from build123d import *

# Parameters (mm, degrees)
F0_W           = 177.8
F0_H           = 228.6
F1_DEPTH       = 12.7
F2_R           = 38.1
F3_DEPTH       = 25.4
F4_SIZE        = 2.54
F5_R           = 5.08
F7_D           = 58.42
F7_CBORE_D     = 63.5
F7_CBORE_DEPTH = 3.175


with BuildPart() as f1:
    # F0 (on Front) → F1 (new body)
    with BuildSketch(Plane.XZ):
        with Locations((88.9, 114.3)):
            Rectangle(F0_W, F0_H)
    extrude(amount=F1_DEPTH)

    # F2 (on face) → F3 (join)
    with BuildSketch(Plane.XZ.offset(12.7)):
        with Locations((63.5, 152.4)):
            Circle(F2_R)
        with Locations((63.5, 63.5)):
            Circle(F2_R)
    extrude(amount=F3_DEPTH)

    # F4
    f4_edges = [f1.edges().sort_by_distance(p)[0] for p in [
        (177.8, -12.7, 114.3),
        (177.8, 0, 114.3),
        (88.9, -12.7, 228.6),
        (88.9, 0, 228.6),
        (0, -12.7, 114.3),
        (0, 0, 114.3),
        (88.9, -12.7, 0),
        (88.9, 0, 0),
        (0, -6.35, 0),
        (177.8, -6.35, 0),
        (0, -6.35, 228.6),
        (177.8, -6.35, 228.6),
    ]]
    chamfer(f4_edges, length=F4_SIZE)

    # F5
    f5_edges = [f1.edges().sort_by_distance(p)[0] for p in [
        (25.4, -38.1, 63.5),
        (25.4, -38.1, 152.4),
    ]]
    fillet(f5_edges, radius=F5_R)

    # F7 (through all)
    with Locations(Plane.XZ.offset(38.1)):
        with Locations((63.5, 152.4), (63.5, 63.500218)):
            CounterBoreHole(F7_D / 2, F7_CBORE_D / 2, F7_CBORE_DEPTH)


solid = f1.part
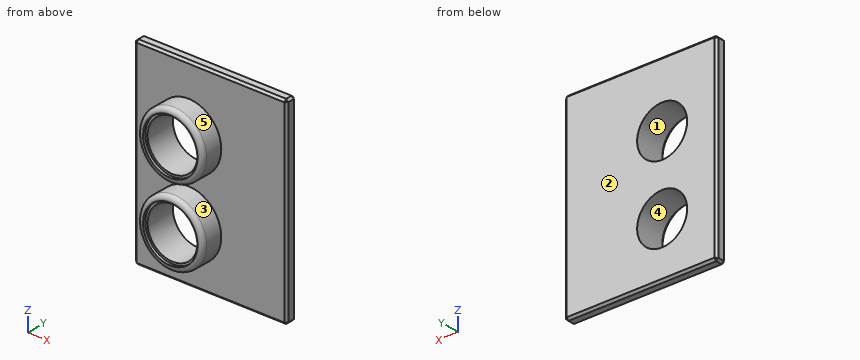
Geometry check sheet. Reference: the model listing, model coordinates, mm. Face numbers are marked on the shaded views. A direction names the side the tool comes from. Round coordinates to 2 decimals unless told otherwise and drop trailing zeros. Write each loop counter-clockwise with the first axis right and the second up, starting at its lowest first coordinate (ties: lowest second). Pieces come first, ordered by that corner, then holes. Notation, with made-up numbers: (77, 0.25) - (136, 0.25) arc R26 cw to (136, 19.25) - close; hole circle Ø5 at (66.5, -7). An arc over 180 degrees is marked (long way). One line per item, written item: value.
1. Cross-section at C-C on y = -26. Record the boundary of the cut face in (x, z), and give its area (3 significant figures).
The answers:
outline: circle Ø76.2 at (63.5, 63.5); circle Ø76.2 at (63.5, 152.4); hole circle Ø58.42 at (63.5, 63.5); hole circle Ø58.42 at (63.5, 152.4)
area: 3,760 mm^2
2. Depth check by flat-ended pin: pin 1 Ø3 at (x, z) = (135.5, 192.5) entering from -Y; pin 2 Ø6 at (x, y) = (60.5, -33.5) entering from +Z; pin 3 Ø2 at (x, y) = (68.5, -12.5) entering from +Z. Enter the tip coordinate at first touch or a pass-through.
The answers:
pin 1: stops at y = -12.7
pin 2: stops at z = 190.5
pin 3: stops at z = 227.26
3. Cross-section at D-D on x = 63.5. Give the number of separate pieces and of enclosed holes in the cut face, and give its area (3 significant figures).
The answers:
separate pieces: 3
enclosed holes: 0
area: 2,260 mm^2
4. Cross-section at A-A on z = 152.4. Record the boundary of the cut face in (x, y) (3 decimals), and give its area (3 significant figures).
The answers:
outline: (0, -10.16) - (2.54, -12.7) - (25.4, -12.7) - (25.4, -33.02) arc R5.08 ccw to (30.48, -38.1) - (31.75, -38.1) - (31.75, -34.925) - (34.29, -34.925) - (34.29, 0) - (2.54, 0) - (0, -2.54) - close; (92.71, -34.925) - (95.25, -34.925) - (95.25, -38.1) - (96.52, -38.1) arc R5.08 ccw to (101.6, -33.02) - (101.6, -12.7) - (175.26, -12.7) - (177.8, -10.16) - (177.8, -2.54) - (175.26, 0) - (92.71, 0) - close
area: 1,930 mm^2
5. Mould release check, pull along X, two halves, no side actions. Record for the marked faces 1, 2 and 3: released by +X, released by -X, zero draft, split by the parting line, or undercut.
The answers:
face 1: undercut
face 2: zero draft
face 3: split by the parting line
6. Scan lines: L1, parallel to Z at x = 63.5, y = -24.5; L2, parallel to X at y = -9, z = 152; L3, parallel to Z at x = 63, y = -36. Record each from-to range of solid material in increasing order.
The answers:
L1: z = 25.4 to 34.29, 92.71 to 101.6, 114.3 to 123.19, 181.61 to 190.5
L2: x = 0 to 34.29, 92.71 to 177.8
L3: z = 26.37 to 31.75, 95.25 to 100.63, 115.27 to 120.65, 184.15 to 189.53
7. Cross-section at B-B on x = 154.5. Record the boundary of the cut face in (y, z), and give its area (3 significant figures).
The answers:
outline: (-12.7, 2.54) - (-10.16, 0) - (-2.54, 0) - (0, 2.54) - (0, 226.06) - (-2.54, 228.6) - (-10.16, 228.6) - (-12.7, 226.06) - close
area: 2,890 mm^2
8. Set-up check for the marked faces 4 and 5: record each of +Z, -Z, +X, -X, +Y, -Y from which the full face is reachable in a straight line by a thin tool's end or side.
The answers:
face 4: +Y, -Y
face 5: -Y
